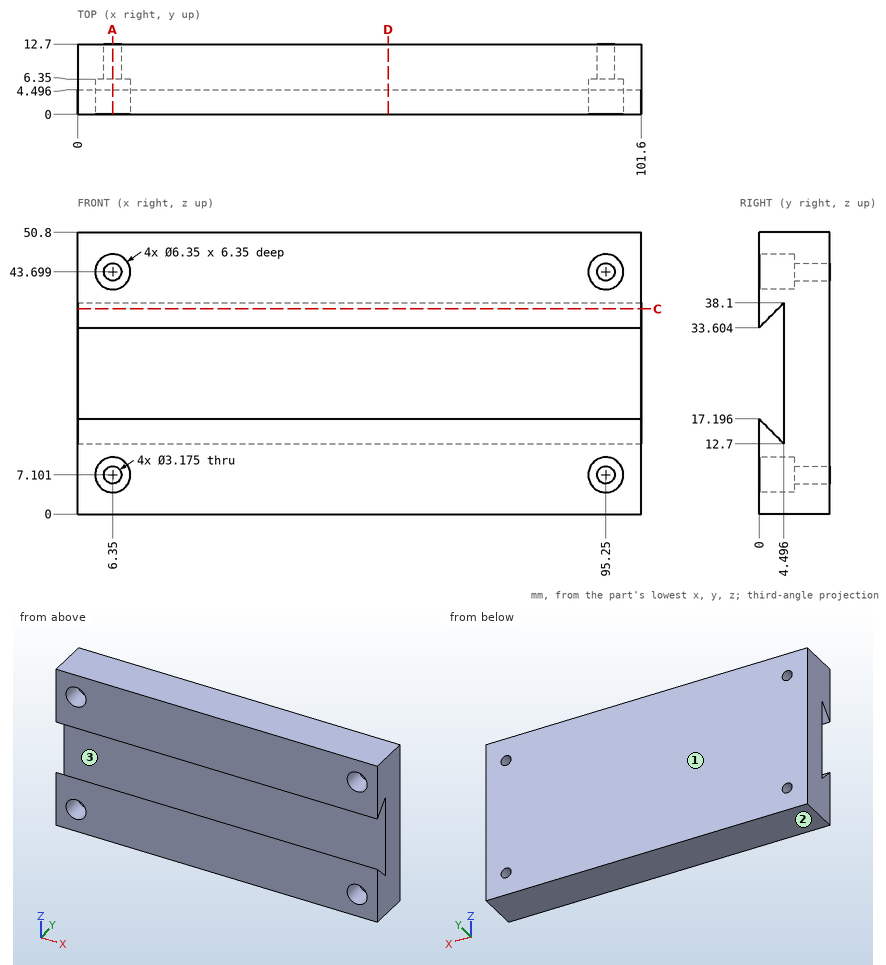
Study the drawing (mm; zero at the part's minimum x, y, z) and answer. Give positions to 0.01 mm unless a question says otherwise; leave off trailing zeros. Loops run counter-clockwise (first coordinate to the right, second up) from the corner with the lowest first, then second, coordinate; pieces in that order, holes last. Notation, with made-up numbers: (58, 81) - (97, 81) arc R22 ccw to (97, 110) - close; hole circle Ø2 at (58, 13). An arc over 180 degrees is marked (long way). Answer as CSV lines item,"result". Start each with the question number.
1) Each of these flat-tipped pins is pushed along its axis until it touches: pin 1 Ø3 at (x, z) = (7.5, 7) entering from -Y; pin 2 Ø5 at (x, z) = (96, 8) entering from -Y. Where does it stop, or does it pass through?
2) Straight lines are drawn through the part: L1, parallel to Z at x = 95.25, y = 11; L2, parallel to Z at x = 95.25, y = 3.25 (1 decimal); L3, parallel to Z at x = 6.35, y = 2.5 (1 decimal). For each, find the intervals that lie inside material, in ascending order. Write a range as from..to.
3) Determine the mould class of the marked faces 1, 2 and 3 for opening direction Y: released by +Y, released by -Y, zero draft, split by the parting line, or undercut.
4) Find section A-A (x = 6.35). State how many separate pieces and enclosed holes the cut face has, then the cut area to 3 significant figures.
5) Find section D-D (x = 56). Write down the section's boundary in (y, z) (1 decimal).
6) Find section C-C (z = 37). Write down the section's boundary in (x, y) (1 decimal).
Findings below:
1,pin 1,"y = 6.35"
1,pin 2,"y = 0"
2,L1,"0..5.51, 8.69..42.11, 45.29..50.8"
2,L2,"0..3.9, 10.3..13.9, 36.9..40.5, 46.9..50.8"
2,L3,"0..3.9, 10.3..14.7, 36.1..40.5, 46.9..50.8"
3,face 1,"released by +Y"
3,face 2,"zero draft"
3,face 3,"undercut"
4,separate pieces,"3"
4,enclosed holes,"0"
4,area,"430 mm^2"
5,outline,"(0, 0) - (12.7, 0) - (12.7, 50.8) - (0, 50.8) - (0, 33.6) - (4.5, 38.1) - (4.5, 12.7) - (0, 17.2) - close"
6,outline,"(0, 0) - (101.6, 0) - (101.6, 3.4) - (0, 3.4) - close; (0, 4.5) - (101.6, 4.5) - (101.6, 12.7) - (0, 12.7) - close"
